from build123d import *

# Parameters (mm, degrees)
CROQUIS2_R              = 7
SALIENTE_EXTRUIR1_DEPTH = 55
CROQUIS3_R              = 12.425
SALIENTE_EXTRUIR2_DEPTH = 20
CROQUIS4_R              = 5
CORTAR_EXTRUIR1_DEPTH   = 47
CROQUIS7_R              = 3
CORTAR_EXTRUIR2_DEPTH   = 8


with BuildPart() as part:
    # Croquis2 → Saliente-Extruir1 (new body)
    with BuildSketch(Plane(origin=(0, 0, 0), x_dir=(1, 0, 0), z_dir=(0, 1, 0))):
        with Locations(Location((0, 0, 0), (0, 0, 270))):
            Circle(CROQUIS2_R)
    extrude(amount=SALIENTE_EXTRUIR1_DEPTH)

    # Croquis3 → Saliente-Extruir2 (add)
    with BuildSketch(Plane(origin=(0, 55, 0), x_dir=(1, 0, 0), z_dir=(0, 1, 0))):
        with Locations(Location((0, 0, 0), (0, 0, 270))):
            Circle(CROQUIS3_R)
    extrude(amount=-SALIENTE_EXTRUIR2_DEPTH)

    # Croquis4 → Cortar-Extruir1 (cut)
    with BuildSketch(Plane(origin=(0, 55, 0), x_dir=(1, 0, 0), z_dir=(0, 1, 0))):
        with Locations(Location((0, 0, 0), (0, 0, 270))):
            Circle(CROQUIS4_R)
    extrude(amount=-CORTAR_EXTRUIR1_DEPTH, mode=Mode.SUBTRACT)

    # Croquis7 → Cortar-Extruir2 (cut)
    with BuildSketch(Plane.XZ):
        with Locations(Location((0, 0, 0), (0, 0, 270))):
            Circle(CROQUIS7_R)
    extrude(amount=-CORTAR_EXTRUIR2_DEPTH, mode=Mode.SUBTRACT)

    # Croquis5 → Cortar-Revolución1 (revolve, cut)
    with BuildSketch(Plane.XY, mode=Mode.PRIVATE) as cortar_revoluci_n1_sk:
        Polygon((-5, 49), (0, 49), (0, 63.271347918), (-20.39383665, 63.271347918), (-20.39383665, 37), (-12.425, 37), (-7, 37), (-7, 39), (-12.425, 39), (-12.425, 41), (-7, 41), (-7, 43), (-12.425, 43), (-12.425, 45), (-7, 45), (-7, 47), (-12.425, 47), (-12.425, 49), (-8.025, 49), (-8.025, 51), (-12.425, 51), (-12.425, 53), (-11.425, 53), (-11.425, 55), (-10, 55), align=None)
    revolve(cortar_revoluci_n1_sk.sketch.rotate(Axis((0, 0, 0), (0, 1, 0)), 270), axis=Axis((0, 0, 0), (0, 1, 0)), mode=Mode.SUBTRACT)


solid = part.part
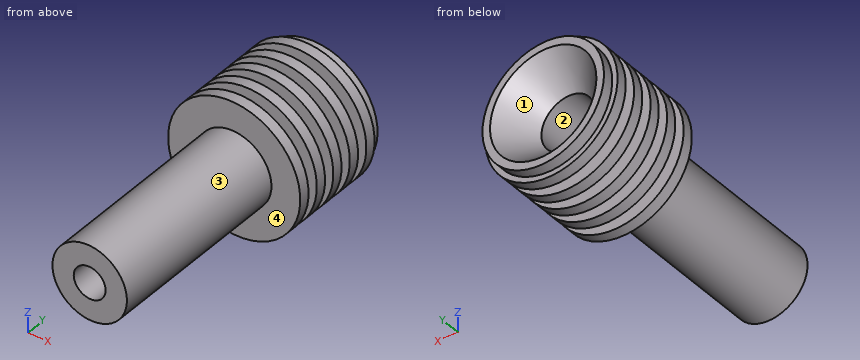
Source: CAD feature listing. Evaluate the final solid. Frame: model axes, mm. Face numbers are marked on the shaded views. Coordinates: 2 decimals unless noted, no trailing zeros. Loops run counter-clockwise (first coordinate to the right, second up) from the corner with the lowest first, then second, coordinate; pieces in that order, holes last. Notation, with made-up numbers: (-33.75, 73) -> (-12.75, 73) arc R15 ccw to (-12.75, 94) -> close; hole circle Ø9 at (-7.75, 1.5). An arc over 180 degrees is marked (long way). Answer in a Markdown table with one row per item. Add a question column.
Q1. Contact query for flat-ended pins moving along their axis: pin 1 Ø8 at (x, y) = (-5.5, 12.5) entering from +Z; pin 2 Ø5 at (x, z) = (0, 0) entering from -Y; pin 3 Ø7.5 at (x, z) = (4, 0.5) entering from +Y; pin 4 Ø8 at (x, y) = (8.5, 42.5) entering from +Z. Output: stop coordinate, or through.
Q2. Ray query, line 1 along Y through (x, z) = (-9.5, 4.5); line 2 along X through (y, z) = (2.75, 0); line 3 along Y through (x, z) = (-3.5, -11). Return the intervals inside material, ascending.
Q3. Section A-A on y = 28. Return the cut outline in (x, z).
Q4. Pull-direction query (Z, two-part tool) for the marked faces 1, 2, 3 and 4; classes: pulls with the +Z half, pulls with the -Z half, needs draft (parallel to the pull), parting line crosses it, or undercut.
Computed values:
| question | item | result |
|---|---|---|
| 1 | pin 1 | stops at z = 6.84 |
| 1 | pin 2 | passes through |
| 1 | pin 3 | stops at y = 52.34 |
| 1 | pin 4 | stops at z = 11.57 |
| 2 | line 1 | y = 35 to 37, 39 to 41, 43 to 45, 47 to 49, 51 to 55 |
| 2 | line 2 | x = -7 to -3, 3 to 7 |
| 2 | line 3 | y = 35 to 37, 39 to 41, 43 to 45, 47 to 49, 51 to 53 |
| 3 | outline | circle Ø14 at (0, 0); hole circle Ø10 at (0, 0) |
| 4 | face 1 | undercut |
| 4 | face 2 | undercut |
| 4 | face 3 | parting line crosses it |
| 4 | face 4 | needs draft |
